from build123d import *

# Parameters (mm, degrees)
SKETCH_1_R          = 14.8
EXTRUDE_1_DEPTH     = 5
SKETCH_2_R          = 17.5
EXTRUDE_2_DEPTH     = 3
SKETCH_3_W          = 10.2
SKETCH_3_H          = 10.2
CUT_EXTRUDE_1_DEPTH = 9
EXTRUDE_3_DEPTH     = 5


with BuildPart() as part:
    # Эскиз1 → Бобышка-Вытянуть1 (new body)
    with BuildSketch(Plane(origin=(0, 0, 0), x_dir=(1, 0, 0), z_dir=(0, 1, 0))):
        with Locations(Location((0, 0, 0), (0, 0, 270))):  # turned: the seam where the file's is
            Circle(SKETCH_1_R)
    extrude(amount=EXTRUDE_1_DEPTH)

    # Эскиз2 → Бобышка-Вытянуть2 (add)
    with BuildSketch(Plane(origin=(0, 5, 0), x_dir=(1, 0, 0), z_dir=(0, 1, 0))):
        with Locations(Location((0, 0, 0), (0, 0, 270))):  # turned: the seam where the file's is
            Circle(SKETCH_2_R)
    extrude(amount=EXTRUDE_2_DEPTH)

    # Эскиз3 → Вырез-Вытянуть1 (cut, through all)
    with BuildSketch(Plane(origin=(0, 8, 0), x_dir=(1, 0, 0), z_dir=(0, 1, 0))):
        Rectangle(SKETCH_3_W, SKETCH_3_H)
    extrude(amount=-CUT_EXTRUDE_1_DEPTH, mode=Mode.SUBTRACT)

    # Эскиз4 → Бобышка-Вытянуть3 (add)
    with BuildSketch(Plane.XZ):
        with BuildLine():
            Line((14.046133482, 4.663275051), (5.1, 1.693185017))
            Line((5.1, 1.693185017), (5.1, -2.944486373))
            Line((5.1, -2.944486373), (12.817175976, -7.4))
            ThreePointArc((12.817175976, -7.4), (14.723790273, -1.5), (14.046133482, 4.663275051))
        make_face()
    extrude(amount=EXTRUDE_3_DEPTH)


solid = part.part
Check sheet for the modelled part. Datum: model origin and axes. Units: mm. A direction names the side the tool comes from. Give positions to 0.01 mm unless a question says otherwise; leave off trailing zeros. Loops run counter-clockwise (first coordinate to the right, second up) from the corner with the lowest first, then second, coordinate; pieces in that order, holes last. Notation, with made-up numbers: M 20,5.25 L 27,5.25 A19 cw 27,18.25 Z; hole C 84.5,32 d3. An arc over 180 degrees is marked long. Answer as a JSON object with one key per item and string values. Group by question number.
Q1. Access from +Z, -Z, +X, -X, +Y, -Y to the whole of each face (thin tool, end or side, straight path). Record for faces 1 (the flat face through (8.9, -2.46, -5.14)), 2 (the flat face through (-8, 8, 0)), 3 (the flat face through (8, 5, -13)), 4 (the flat face through (-5.1, 4, 0)).
Q2. Release check for a two-part mould opening along X. For faces 5 (the flat face through (5.1, 3, 0)), 6 (the flat face through (-7, 0, 0)), 7 (the flat face through (9.64, -2.46, 3.2)) record: released by +X, released by -X, zero draft, split by the parting line, or undercut.
Q3. Go/stop test with flat-tipped pins: P1, Ø2, axis at x = 10, y = 3, coming from the -Z side; P2, Ø3, axis at y = 2.5, z = -10, coming from the -X side; P3, Ø4, axis at x = 11, z = -9, coming from the -Y side. Record where each tip stops, or that it passes through.
Q4. Cross-section at A-A on x = 0. Record the cut outline in (y, z).
Q5. Cross-section at B-B on z = 0. Record the cut outline in (x, y), then the cut area to 3 significant figures.
Q6. Material ranges on line 1 along Y through (x, z) = (-0.5, 6); line 2 along Z through (x, y) = (2, 6.25); line 3 along Z through (x, y) = (1.5, 1.25), recorded low to high. Write a range as [from, to].
Q7. Cross-section at C-C on x = -14. Record the cut outline in (y, z).
Q8. Cross-section at D-D on y = 0.5. Record the cut outline in (x, z), then the cut area to 3 significant figures.
Evaluation:
{
 "1": {"face 1": "-Z, -X, -Y", "face 2": "+Z, -Z, +X, -X, +Y", "face 3": "-Y", "face 4": "+Y, -Y"},
 "2": {"face 5": "undercut", "face 6": "zero draft", "face 7": "released by -X"},
 "3": {"P1": "stops at z = -11.75", "P2": "stops at x = -12.12", "P3": "stops at y = 0"},
 "4": {"outline": "M 0,-14.8 L 5,-14.8 L 5,-17.5 L 8,-17.5 L 8,-5.1 L 0,-5.1 Z; M 0,5.1 L 8,5.1 L 8,17.5 L 5,17.5 L 5,14.8 L 0,14.8 Z"},
 "5": {"outline": "M -17.5,5 L -14.8,5 L -14.8,0 L -5.1,0 L -5.1,8 L -17.5,8 Z; M 5.1,-5 L 14.8,-5 L 14.8,5 L 17.5,5 L 17.5,8 L 5.1,8 Z", "area": "220 mm2"},
 "6": {"line 1": "y = [0, 8]", "line 2": "z = [-17.39, -5.1], [5.1, 17.39]", "line 3": "z = [-14.72, -5.1], [5.1, 14.72]"},
 "7": {"outline": "M 0,-4.8 L 5,-4.8 L 5,-10.5 L 8,-10.5 L 8,10.5 L 5,10.5 L 5,4.8 L 0,4.8 Z"},
 "8": {"outline": "C 0,0 d29.6; hole M -5.1,-5.1 L 5.1,-5.1 L 5.1,5.1 L -5.1,5.1 Z", "area": "584 mm2"}
}
